from build123d import *

# Parameters (mm, degrees)
F0_W        = 127
F0_H        = 76.2
F1_DEPTH    = 12.7
F2_R        = 6.35
F3_DEPTH    = 12.701
F4_W        = 12.7
F4_H        = 50.8
F6_W        = 7.62
F6_H        = 12.7
F8_R        = 5.08
F9_T1_DEPTH = 153.1282991577
F9_T3_DEPTH = 102.3282991577


# Not quite as in the source:
# - a fillet or chamfer that OpenCascade refuses, or shapes differently, is made with other operations: its cross-section is extruded or revolved along the edge and cut away or added


with BuildPart() as f1:
    # F0 (on Top) → F1 (new body)
    with BuildSketch(Plane.XY):
        Rectangle(F0_W, F0_H)
    extrude(amount=F1_DEPTH)

    # F2 (on face) → F3 (cut, through all)
    with BuildSketch(Plane.XY.offset(12.7)):
        with Locations((-39.8141870437, -23.5891287784)):
            Circle(F2_R)
        with Locations((47.751432499, 20.7712577737)):
            Circle(F2_R)
        with Locations((-39.8141870437, 19.3517001108)):
            Circle(F2_R)
        with Locations((50.5741164088, -27.9485974461)):
            Circle(F2_R)
    extrude(amount=-F3_DEPTH, mode=Mode.SUBTRACT)

    # F4 (on Front) → F5 (revolve)
    with BuildSketch(Plane.XZ):
        with Locations((6.35, 38.1)):
            Rectangle(F4_W, F4_H)
    revolve(axis=Axis((0, 0, 38.1), (0, 0, 1)))

    # F6 (on Front) → F7 (revolve, cut)
    with BuildSketch(Plane.XZ):
        with Locations((10.6961938009, 36.2604726106)):
            Rectangle(F6_W, F6_H)
    revolve(axis=Axis((0, 0, 12.7), (0, 0, 1)), mode=Mode.SUBTRACT)

    # F8
    f8_edges = [f1.edges().sort_by_distance(p)[0] for p in [
        (-12.7, 0, 29.910473),
        (-12.7, 0, 63.5),
        (-12.7, 0, 12.7),
    ]]
    fillet(f8_edges, radius=F8_R)

    # F9: chamfer of 5.08 on 7 edges, made by hand

    # F9_s2 → F9_t1 (cut)
    with BuildSketch(Plane.YZ.offset(-76.5641495789)):
        Polygon((33.02, 12.7), (38.1, 7.62), (38.1, 12.7), align=None)
        Polygon((-33.02, 12.7), (-38.1, 7.62), (-38.1, 12.7), align=None)
    extrude(amount=F9_T1_DEPTH, mode=Mode.SUBTRACT)

    # F9_s4 → F9_t3 (cut)
    with BuildSketch(Plane.XZ.offset(-51.1641495789)):
        Polygon((58.42, 12.7), (63.5, 7.62), (63.5, 12.7), align=None)
        Polygon((-58.42, 12.7), (-63.5, 7.62), (-63.5, 12.7), align=None)
    extrude(amount=F9_T3_DEPTH, mode=Mode.SUBTRACT)


solid = f1.part
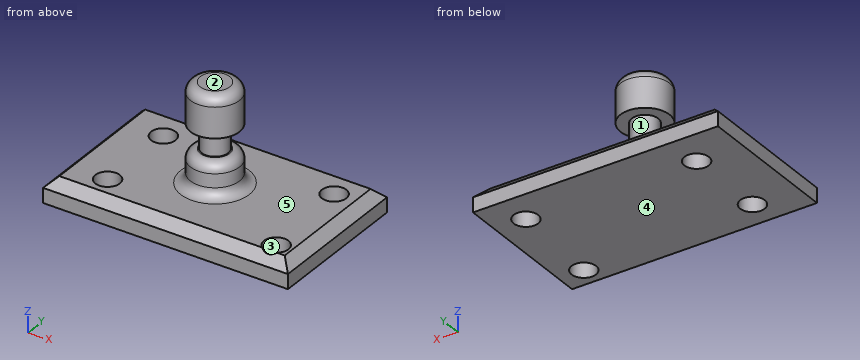
Input: part model. Units: mm. Frame: model coordinates. Face numbers are marked on the shaded views. A direction names the side the tool comes from. Round coordinates to 2 decimals unless told otherwise and drop trailing zeros. Order: outer loops, then holes, each group sorted by start corner. A loop starts at its lowest first (then second) coordinate and runs counter-clockwise, first axis right, second up. Notation, with made-up numbers: (-27, -31) - (19, -31) arc R23 ccw to (19, -11) - close; hole circle Ø10 at (67, 46.5). An arc over 180 degrees is marked (long way). Use a Markdown table: item, result.
1. First-contact query: pin 1 (3 mm diameter, centred on x = 24, y = 17.5, fed in from -Z); pin 2 (14.5 mm diameter, centred on x = 50.57, y = -27.95, fed in from +Z); pin 3 (7.5 mm diameter, centred on x = -39.81, y = -23.59, fed in from +Z) (3 decimals). Flat tips, straight axial feed; report the tip coordinate or a pass-through.
Evaluation:
| item | result |
|---|---|
| pin 1 | z = 0 |
| pin 2 | z = 12.7 |
| pin 3 | through |
2. Mould query, pull axis Y, two halves, no side actions, for the marked faces 1, 2 and 3. Classes: +Y half, -Y half, draft (parallel to the pull), parting line (faces both ways), or undercut.
Evaluation:
| item | result |
|---|---|
| face 1 | parting line |
| face 2 | draft |
| face 3 | undercut |
3. Section D-D on x = 0. Return the cut outline in (y, z).
Evaluation:
| item | result |
|---|---|
| outline | (-38.1, 0) - (38.1, 0) - (38.1, 7.62) - (33.02, 12.7) - (17.78, 12.7) arc R5.08 cw to (12.7, 17.78) - (12.7, 24.83) arc R5.08 ccw to (7.62, 29.91) - (6.89, 29.91) - (6.89, 42.61) - (12.7, 42.61) - (12.7, 58.42) arc R5.08 ccw to (7.62, 63.5) - (-7.62, 63.5) arc R5.08 ccw to (-12.7, 58.42) - (-12.7, 42.61) - (-6.89, 42.61) - (-6.89, 29.91) - (-7.62, 29.91) arc R5.08 ccw to (-12.7, 24.83) - (-12.7, 17.78) arc R5.08 cw to (-17.78, 12.7) - (-33.02, 12.7) - (-38.1, 7.62) - close |
4. Material intervals for probe 1 along X at (y, z) = (-23.5, 7.5); probe 2 along X at (y, z) = (16.5, 4); probe 3 along Z at (x, y) = (3.5, -18.5), sorted ascending.
Evaluation:
| item | result |
|---|---|
| probe 1 | -63.5 to -46.16, -33.46 to 46.04, 55.11 to 63.5 |
| probe 2 | -63.5 to -45.49, -34.14 to 43.05, 52.45 to 63.5 |
| probe 3 | 0 to 12.7 |
5. Access query for the marked faces 4 and 5. Directions: +Z, -Z, +X, -X, +Y, -Y. A direction counts if a zero-diameter tool reaches every point of the face in a straight line with its end or side. Return the directions, or none.
Evaluation:
| item | result |
|---|---|
| face 4 | -Z, +X, -X, +Y, -Y |
| face 5 | +Z |
6. Section A-A on z = 6. Return the cut outline in (x, y).
Evaluation:
| item | result |
|---|---|
| outline | (-63.5, -38.1) - (63.5, -38.1) - (63.5, 38.1) - (-63.5, 38.1) - close; hole circle Ø12.7 at (-39.81, -23.59); hole circle Ø12.7 at (-39.81, 19.35); hole circle Ø12.7 at (47.75, 20.77); hole circle Ø12.7 at (50.57, -27.95) |
7. Section B-B on x = -35. Return the cut outline in (y, z).
Evaluation:
| item | result |
|---|---|
| outline | (-38.1, 0) - (-27.73, 0) - (-27.73, 12.7) - (-33.02, 12.7) - (-38.1, 7.62) - close; (-19.45, 0) - (15.21, 0) - (15.21, 12.7) - (-19.45, 12.7) - close; (23.49, 0) - (38.1, 0) - (38.1, 7.62) - (33.02, 12.7) - (23.49, 12.7) - close |
8. Section C-C on y = 0. Return the cut outline in (x, z), then the cut area to 3 significant figures.
Evaluation:
| item | result |
|---|---|
| outline | (-63.5, 0) - (63.5, 0) - (63.5, 7.62) - (58.42, 12.7) - (17.78, 12.7) arc R5.08 cw to (12.7, 17.78) - (12.7, 24.83) arc R5.08 ccw to (7.62, 29.91) - (6.89, 29.91) - (6.89, 42.61) - (12.7, 42.61) - (12.7, 58.42) arc R5.08 ccw to (7.62, 63.5) - (-7.62, 63.5) arc R5.08 ccw to (-12.7, 58.42) - (-12.7, 42.61) - (-6.89, 42.61) - (-6.89, 29.91) - (-7.62, 29.91) arc R5.08 ccw to (-12.7, 24.83) - (-12.7, 17.78) arc R5.08 cw to (-17.78, 12.7) - (-58.42, 12.7) - (-63.5, 7.62) - close |
| area | 2,720 mm^2 |
